Autodesk Inventor part; units mm, degrees
ref_plane "YZ Plane" through (0, 0, 0) normal (1, 0, 0) x (0, 1, 0)
ref_plane "XZ Plane" through (0, 0, 0) normal (0, 1, 0) x (-1, 0, 0)
ref_plane "XY Plane" through (0, 0, 0) normal (0, 0, 1) x (1, 0, 0)
sketch "スケッチ1" plane through (0, 0, 0) normal (0, 0, 1) x (1, 0, 0)
  line L0 (5.096, 0) -> (-5.096, 0) construction
  circle A0 centre (20, 15) radius 4
  circle A1 centre (20, 15) radius 8
  circle A2 centre (20, 15) radius 6 construction
  circle A3 centre (20, 21) radius 1.1
  circle A4 centre (15.7574, 19.2426) radius 1.1
  circle A5 centre (14, 15) radius 1.1
  circle A6 centre (15.7574, 10.7574) radius 1.1
  circle A7 centre (20, 9) radius 1.1
  circle A8 centre (24.2426, 10.7574) radius 1.1
  circle A9 centre (26, 15) radius 1.1
  circle A10 centre (24.2426, 19.2426) radius 1.1
  circle A11 centre (-10, 0) radius 1.6
  circle A12 centre (20, -15) radius 4
  circle A13 centre (20, -15) radius 8
  circle A14 centre (20, -15) radius 6 construction
  circle A15 centre (20, -21) radius 1.1
  circle A16 centre (15.7574, -19.2426) radius 1.1
  circle A17 centre (14, -15) radius 1.1
  circle A18 centre (15.7574, -10.7574) radius 1.1
  circle A19 centre (20, -9) radius 1.1
  circle A20 centre (24.2426, -10.7574) radius 1.1
  circle A21 centre (26, -15) radius 1.1
  circle A22 centre (24.2426, -19.2426) radius 1.1
  circle A23 centre (-10, 0) radius 1.6
  circle A24 centre (-10, 0) radius 3.5
  circle A25 centre (-10, 0) radius 3.5
  line L1 (-11.6951, 3.0621) -> (13.0314, 16.7498)
  line L2 (28, 15) -> (28, -15)
  circle A26 centre (14, 15) radius 2
  circle A27 centre (26, 15) radius 2
  line L3 (-11.6951, -3.0621) -> (13.0314, -16.7498)
  circle A28 centre (14, -15) radius 2
  circle A29 centre (26, -15) radius 2
  line L4 (-13.5, 0) -> (-13.5, 0)
  point P0 (0, 0)
  point P1 (0, 0)
  point P2 (12.0954, 16.2317)
  point P3 (12.0954, -16.2317)
  point P4 (28, -15)
  point P5 (28, 15)
  point P6 (24, 15)
  point P7 (16, 15)
  point P8 (-11.6951, -3.0621)
  point P9 (12.0954, -16.2317)
  point P10 (12, -15)
  point P11 (16, -15)
  point P12 (24, -15)
  dimension "d2" = 12
  dimension "d0" = 8
  dimension "d1" = 16
  dimension "d3" = 2.2
  dimension "d6" = 360
  dimension "d9" = 3.2
  dimension "d10" = 30
  dimension "d11" = 15
  dimension "d12" = 20
  dimension "d13" = 7
extrude "押し出し1" add sketch "スケッチ1" along normal blind 1.5 contours A27 A1 A26 A0 | A27 | A26 | L2 A13 L3 A24 L1 A1 | A26 A1 L1 | A29 A12 A28 A13 | A29 | A24 | A28 L3 A13 | A28
sketch "スケッチ3" plane through (0, 0, 0) normal (0, 0, -1) x (-1, 0, 0)
  arc A0 (-24, 15) -> (-28, 15) centre (-26, 15) ccw
  line L0 (-28, -15) -> (-28, 15)
  arc A1 (-28, -15) -> (-24, -15) centre (-26, -15) ccw
  arc A2 (-16, -15) -> (-24, -15) centre (-20, -15) ccw
  arc A3 (-16, -15) -> (-13.0314, -16.7498) centre (-14, -15) ccw
  line L1 (11.6951, -3.0621) -> (-13.0314, -16.7498)
  arc A4 (11.6951, -3.0621) -> (11.6951, 3.0621) centre (10, 0) ccw
  line L2 (-13.0314, 16.7498) -> (11.6951, 3.0621)
  arc A5 (-13.0314, 16.7498) -> (-16, 15) centre (-14, 15) ccw
  arc A6 (-24, 15) -> (-16, 15) centre (-20, 15) ccw
  circle A7 centre (-14, 15) radius 1.1
  circle A8 centre (-26, 15) radius 1.1
  circle A9 centre (-14, -15) radius 1.1
  circle A10 centre (-26, -15) radius 1.1
  circle A11 centre (-24.2426, -10.7574) radius 1.1
  circle A12 centre (-20, -9) radius 1.1
  circle A13 centre (-15.7574, -10.7574) radius 1.1
  circle A14 centre (10, 0) radius 1.6
  circle A15 centre (-24.2426, 10.7574) radius 1.1
  circle A16 centre (-20, 9) radius 1.1
  circle A17 centre (-15.7574, 10.7574) radius 1.1
  circle A18 centre (-20, 15) radius 8
  circle A19 centre (-20, -15) radius 8
  circle A20 centre (10, 0) radius 3.5
  arc A21 (10.7265, -1.3123) -> (10.7265, 1.3123) centre (10, 0) ccw
  line L3 (10.7265, -1.3123) -> (-14, -15)
  arc A22 (-14, -15) -> (-26, -15) centre (-20, -15) ccw
  line L4 (-26, -15) -> (-26, 15)
  arc A23 (-26, 15) -> (-14, 15) centre (-20, 15) ccw
  line L5 (-14, 15) -> (10.7265, 1.3123)
  line L6 (-26, 0) -> (10, 0) construction
  circle A24 centre (-8, 0) radius 5
  circle A25 centre (-8, 0) radius 6
  line L7 (-26, -0.5) -> (10, -0.5)
  line L8 (10, -0.5) -> (10, 0.5)
  line L9 (10, 0.5) -> (-26, 0.5)
  line L10 (-26, 0.5) -> (-26, -0.5)
  line L11 (-26, -0.5) -> (10, 0.5) construction
  line L12 (10, -0.5) -> (-26, 0.5) construction
  line L13 (4.3904, 14.6877) -> (-19.6096, -15.3123)
  line L14 (-19.6096, -15.3123) -> (-20.3904, -14.6877)
  line L15 (-20.3904, -14.6877) -> (3.6096, 15.3123)
  line L16 (3.6096, 15.3123) -> (4.3904, 14.6877)
  line L17 (4.3904, 14.6877) -> (-20.3904, -14.6877) construction
  line L18 (-19.6096, -15.3123) -> (3.6096, 15.3123) construction
  line L19 (4.3904, -14.6877) -> (-19.6096, 15.3123)
  line L20 (-20.3904, 14.6877) -> (3.6096, -15.3123)
  point P0 (0, 0)
  point P1 (-3.8744, -4.3566)
  point P2 (-1.0809, -7.8485)
  point P3 (7.9598, -2.8439)
  point P4 (6.5359, -0.5)
  point P5 (-2.0209, -0.5)
  point P6 (-14.6218, 9.0776)
  point P7 (-11.3447, 4.9813)
  point P8 (-4.6553, 4.9813)
  point P9 (-1.9685, 8.3398)
  point P10 (-12.0715, 13.9325)
  point P11 (-1.0809, 7.8485)
  point P12 (-3.8744, 4.3566)
  point P13 (-2.0209, 0.5)
  point P14 (6.5359, 0.5)
  point P15 (7.9598, 2.8439)
  point P16 (-1.9685, -8.3398)
  point P17 (-4.6553, -4.9813)
  point P18 (-11.3447, -4.9813)
  point P19 (-14.6218, -9.0776)
  point P20 (-12.0715, -13.9325)
  point P21 (-15.4026, -8.4529)
  point P22 (-12.1256, -4.3566)
  point P23 (-13.9791, -0.5)
  point P24 (-26, -9.7085)
  point P25 (-12.1256, 4.3566)
  point P26 (-15.4026, 8.4529)
  point P27 (-26, 9.7085)
  point P28 (-13.9791, 0.5)
  dimension "d27" = 2
  dimension "d28" = 10
  dimension "d29" = 12
  dimension "d30" = 1
  dimension "d31" = 1
extrude "押し出し3" cut sketch "スケッチ3" against normal through all contours A18 L20 A25 L9 L4 | L4 L7 A25 L15 A19 | L15 A25 L19 A18 L5 | L13 A25 L20 L3 A19 | L5 A20 L9 A25 L13 | L20 L9 A24 | A24 L19 L15 L9 L20 | L9 L20 L15 L7 A24 | L15 L7 L20 L13 A24 | A24 L7 L15 | L19 A25 L7 A20 L3 | L15 L19 A24 | A24 L13 L9 L19 L15 | L9 L15 L20 | L13 L20 A24 | L15 L20 L7 | L20 L13 L7 L19 A24 | A24 L9 L13 | L19 L9 L15 | L9 L19 L13 L7 L20 L15 | L20 L7 L13 | L19 L7 A24 | A24 L7 L19 L13 L9 | L13 L19 L9 | L13 L19 L7
fillet "フィレット2" radius 2 29 edges at (26, -0.5, 0.75) (26, 0.5, 0.75) (13.9791, -0.5, 0.75) (13.9791, 0.5, 0.75) (26, -9.7085, 0.75) (15.4026, -8.4529, 0.75) (12.1256, -4.3566, 0.75) (11.3447, -4.9813, 0.75) (14.6218, -9.0776, 0.75) (12.0715, -13.9325, 0.75) (1.9685, -8.3398, 0.75) (1.0809, -7.8485, 0.75) (4.6553, -4.9813, 0.75) (3.8744, -4.3566, 0.75) (2.0209, -0.5, 0.75) (2.0209, 0.5, 0.75) (-6.5359, -0.5, 0.75) (-7.9598, -2.8439, 0.75) (-7.9598, 2.8439, 0.75) (1.0809, 7.8485, 0.75) (3.8744, 4.3566, 0.75) (4.6553, 4.9813, 0.75) (1.9685, 8.3398, 0.75) (11.3447, 4.9813, 0.75) (14.6218, 9.0776, 0.75) (15.4026, 8.4529, 0.75) (12.1256, 4.3566, 0.75) (26, 9.7085, 0.75) (12.0715, 13.9325, 0.75)
properties part number "hiza" material "アルミニウム 2014-T4"
For this review, take the finished solid that the model builds, in its own axes (mm). A direction names the side the tool comes from. Coordinates: 2 decimals unless noted, no trailing zeros. Write each loop counter-clockwise with the first axis right and the second up, starting at its lowest first coordinate (ties: lowest second). Pieces come first, ordered by that corner, then holes. Notation, with made-up numbers: (3, 61) -> (20, 61) arc R10 ccw to (20, 80) -> close; hole circle Ø1 at (-9, 81.25). An arc over 180 degrees is marked (long way). Put each result on its own line as item: value.
Q1. Take a section at D-D, the plane x = -1. State the section outline as (y, z) points.
From the geometry:
outline: (-8.98, 0) -> (-6.7, 0) -> (-6.7, 1.5) -> (-8.98, 1.5) -> close; (-0.5, 0) -> (0.5, 0) -> (0.5, 1.5) -> (-0.5, 1.5) -> close; (6.7, 0) -> (8.98, 0) -> (8.98, 1.5) -> (6.7, 1.5) -> close
Q2. Take a section at C-C, the plane x = 8. State the section outline as (y, z) points, then the cut area to 3 significant figures.
From the geometry:
outline: (-13.96, 0) -> (-11.68, 0) -> (-11.68, 1.5) -> (-13.96, 1.5) -> close; (-6, 0) -> (-5, 0) -> (-5, 1.5) -> (-6, 1.5) -> close; (5, 0) -> (6, 0) -> (6, 1.5) -> (5, 1.5) -> close; (11.68, 0) -> (13.96, 0) -> (13.96, 1.5) -> (11.68, 1.5) -> close
area: 9.86 mm2
Q3. The part is to be moulded in two halves that separate along X. For faces 1 (the cylindrical face through (24.75, 11.733, 0.74)), 2 (the flat face through (13, -2, 0)), 3 (the cylindrical face through (-13.5, -0.1, 0.7)), say which applies: +X half, -X half, draft (parallel to the pull), parting line (faces both ways), or undercut.
From the geometry:
face 1: undercut
face 2: draft
face 3: -X half
Q4. Tool access review of faces 4 (the cylindrical face through (14, 9, 1)), 5 (the flat face through (0.495, 9.81, 0.74)): name each direction out of +Z, -Z, +X, -X, +Y, -Y from which nothing blocks a thin tool from reaching the whole face with its end or side.
From the geometry:
face 4: +Z, -Z
face 5: +Z, -Z, -X, +Y
Q5. Take a section at A-A, the plane x = 20. State the section outline as (y, z) points, then the cut area to 3 significant figures.
From the geometry:
outline: (-11, 0) -> (-10.1, 0) -> (-10.1, 1.5) -> (-11, 1.5) -> close; (-7.9, 0) -> (-7, 0) -> (-7, 1.5) -> (-7.9, 1.5) -> close; (-0.5, 0) -> (0.5, 0) -> (0.5, 1.5) -> (-0.5, 1.5) -> close; (7, 0) -> (7.9, 0) -> (7.9, 1.5) -> (7, 1.5) -> close; (10.1, 0) -> (11, 0) -> (11, 1.5) -> (10.1, 1.5) -> close
area: 6.90 mm2
Q6. Take a section at B-B, the plane y = -8.5. State the section outline as (x, z) points.
From the geometry:
outline: (-1.87, 0) -> (3.16, 0) -> (3.16, 1.5) -> (-1.87, 1.5) -> close; (13.94, 0) -> (19.02, 0) -> (19.02, 1.5) -> (13.94, 1.5) -> close; (20.98, 0) -> (28, 0) -> (28, 1.5) -> (20.98, 1.5) -> close
Q7. Wall thickness on L1, parallel to Y at x = 8.5, z = 0.3; L2, parallel to Y at x = 15.5, z = 0.65; L3, parallel to Y at x = -5.5, z = 0.7: over which ranges is each line inside the solid? List them lowest first.
From the geometry:
L1: y = -14.24 to -11.96, -5.98 to -4.97, 4.97 to 5.98, 11.96 to 14.24
L2: y = -16.32 to -11.83, -9.69 to -7.84, -0.5 to 0.5, 7.84 to 9.69, 11.83 to 16.32
L3: y = -6.49 to -4.2, -0.79 to 0.5, 4.21 to 6.49
